Part model, mm, in its own coordinate system. A direction names the side the tool comes from. Round coordinates to 2 decimals unless told otherwise and drop trailing zeros. Loops run counter-clockwise (first coordinate to the right, second up) from the corner with the lowest first, then second, coordinate; pieces in that order, holes last. Notation, with made-up numbers: M 34,-1 L 42,-1 A34 cw 42,31 Z; hole C 24.5,26 d1. An arc over 180 degrees is marked long. Put each result on its own line as item: value. Start each with the question number.
1) Slice it at B-B on x = 2.1. Give the cut face in (y, z).
2) Probe line 1 along X through (y, z) = (1.75, 1.3); line 2 along Z through (x, y) = (1.5, 5.5); line 3 along Z through (x, y) = (1.8, 2). List the from-to ranges inside material, lowest first.
3) Drop flat-ended pins along their axis: pin 1 Ø1 at (x, y) = (1.5, 1.5) entering from +Z; pin 2 Ø2.5 at (y, z) = (4, 1.5) entering from +X. Give the stop position or say it passes through.
4) Which spindle directions (+Z, -Z, +X, -X, +Y, -Y) get a long thin tool onto all of the face, cutting with end or side? Do faces 4 (the flat face through (1.588, 3, 2)), 5 (the flat face through (1, 3, 0)). Say none if no direction does.
5) Pull direction X, two halves, no side cores. Call faces 1 (the flat face through (1, 0, 2)), 2 (the flat face through (1.6, 3.13, 4.09)), 3 (the flat face through (0, 3, 2)): +X half, -X half, draft (parallel to the pull), parting line (faces both ways), or undercut.
6) Slice it at C-C on z = 3.05. Give the cut face in (x, y), then the cut area to 3 significant figures.
```python
from build123d import *

# Parameters (mm, degrees)
F0_W     = 6.35
F0_H     = 3.175
F1_DEPTH = 1.5875
F2_W     = 6.35
F2_H     = 1.5875
F3_DEPTH = 2.54
F4_SIZE2 = 1.27
F4_SIZE  = 1.905


with BuildPart() as f1:
    # F0 (on Right) → F1 (new body)
    with BuildSketch(Plane.YZ):
        with Locations((3.175, 1.5875)):
            Rectangle(F0_W, F0_H)
    extrude(amount=F1_DEPTH)

    # F2 (on Right) → F3 (join)
    with BuildSketch(Plane.YZ):
        with Locations((3.175, 3.9399821234)):
            Rectangle(F2_W, F2_H)
    extrude(amount=F3_DEPTH)

    # F4
    f4_edges = [f1.edges().sort_by_distance(p)[0] for p in [
        (2.54, 3.175, 4.733732),
    ]]
    f4_side = f1.faces().sort_by_distance((1.27, 3.175, 4.733732))[0]
    chamfer(f4_edges, length=F4_SIZE, length2=F4_SIZE2, reference=f4_side)


solid = f1.part
```
Recorded:
1. outline: M 0,3.15 L 6.35,3.15 L 6.35,3.76 L 0,3.76 Z
2. line 1: x = 0 to 1.59
2. line 2: z = 0 to 4.16
2. line 3: z = 3.15 to 3.96
3. pin 1: stops at z = 4.49
3. pin 2: stops at x = 1.59
4. face 4: -Z, +X, +Y, -Y
4. face 5: -Z, +X, -X, +Y, -Y
5. face 1: draft
5. face 2: +X half
5. face 3: -X half
6. outline: M 0,0 L 1.59,0 L 1.59,6.35 L 0,6.35 Z
6. area: 10.1 mm2
